from build123d import *

# Parameters (mm, degrees)
SKETCH1_W           = 157.13579329
SKETCH1_H           = 157.13579329
BOSS_EXTRUDE1_DEPTH = 25.4
SKETCH2_W           = 136.81579329
SKETCH2_H           = 111.41579329
CUT_EXTRUDE1_DEPTH  = 22.86
SKETCH3_W           = 136.81579329
SKETCH3_H           = 25.4
CUT_EXTRUDE2_DEPTH  = 22.86
SKETCH5_W           = 5.08
SKETCH5_H           = 136.81579329
CUT_EXTRUDE3_DEPTH  = 7.62
SKETCH6_W           = 8.486375486
SKETCH6_H           = 6.062880986
CUT_EXTRUDE4_DEPTH  = 15.24
SKETCH8_R           = 15.547206761
BOSS_EXTRUDE3_DEPTH = 17.78


with BuildPart() as part:
    # Sketch1 → Boss-Extrude1 (new body)
    with BuildSketch(Plane.XY):
        Rectangle(SKETCH1_W, SKETCH1_H)
    extrude(amount=BOSS_EXTRUDE1_DEPTH)

    # Sketch2 → Cut-Extrude1 (cut)
    with BuildSketch(Plane.XY.offset(25.4)):
        with Locations((0, 12.7)):
            Rectangle(SKETCH2_W, SKETCH2_H)
    extrude(amount=-CUT_EXTRUDE1_DEPTH, mode=Mode.SUBTRACT)

    # Sketch3 → Cut-Extrude2 (cut)
    with BuildSketch(Plane.XY.offset(25.4)):
        with Locations((0, -60.787896645)):
            Rectangle(SKETCH3_W, SKETCH3_H)
    extrude(amount=-CUT_EXTRUDE2_DEPTH, mode=Mode.SUBTRACT)

    # Sketch5 → Cut-Extrude3 (cut)
    with BuildSketch(Plane.ZY.offset(78.567896645)):
        with Locations((12.7, 0)):
            Rectangle(SKETCH5_W, SKETCH5_H)
    cut_extrude3 = extrude(amount=-CUT_EXTRUDE3_DEPTH, mode=Mode.SUBTRACT)

    # Mirror1: Cut-Extrude3 across plane
    add(cut_extrude3.mirror(Plane(origin=(0, 0, 0), x_dir=(0, 0, 1), z_dir=(1, 0, 0))), mode=Mode.SUBTRACT)

    # Sketch6 → Cut-Extrude4 (cut)
    with BuildSketch(Plane.XY.offset(25.4)):
        with Locations((-51.293944562, 71.439337138)):
            Rectangle(SKETCH6_W, SKETCH6_H)
    extrude(amount=-CUT_EXTRUDE4_DEPTH, mode=Mode.SUBTRACT)

    # Sketch8 → Boss-Extrude3 (add)
    with BuildSketch(Plane.XY.offset(2.54)):
        with Locations((39.391283746, 8.898945532)):
            Circle(SKETCH8_R)
    extrude(amount=BOSS_EXTRUDE3_DEPTH)


solid = part.part
Verification items for the finished model (mm, model axes). A direction names the side the tool comes from. Round coordinates to 2 decimals unless told otherwise and drop trailing zeros. Loops run counter-clockwise (first coordinate to the right, second up) from the corner with the lowest first, then second, coordinate; pieces in that order, holes last. Notation, with made-up numbers: (43.25, 37.5) - (53.25, 37.5) arc R36 ccw to (53.25, 71.5) - close; hole circle Ø3 at (-10.5, -9.5). An arc over 180 degrees is marked (long way). Answer in a Markdown table with one row per item. Add a question column.
Q1. Gauge pin test, flat ends, axial feed: pin 1 (10 mm diameter, centred on x = 13.5, y = -24.5, fed in from +Z); pin 2 (15.5 mm diameter, centred on x = 41.5, y = 2.5, fed in from +Z). Record the tip position at first contact, or that the pin passes through.
Q2. Release check for a two-part mould opening along Z. For faces 4 (the face through (-1, -78.568, 13)), 5 (the face through (-1, 13, 2.54)), 6 (the face through (75, -1, 15.24)), 7 (the face through (-75, -1, 10.16)) record: pulls with the +Z half, pulls with the -Z half, needs draft (parallel to the pull), parting line crosses it, or undercut.
Q3. Section check C-C on y = -45. Enter the section's corners in (x, z), plus the area to 3 significant figures.
Q4. Section check B-B on x = -49. Enter the section's corners in (y, z), plus the area to 3 significant figures.
Q5. Section check D-D on y = 38. Enter the section's corners in (x, z), plus the area to 3 significant figures.
Q6. Material ranges on line 1 (Y direction, x = 17, z = 8.75); line 2 (X direction, y = -58, z = 18.75); line 3 (X direction, y = 14.5, z = 15), recorded low to high.
Q7. Section check A-A on z = 17.75. Enter the section's corners in (x, y), plus the area to 3 significant figures.
Q8. Tool access check on faces 1 (the face through (68.408, -61, 14)), 2 (the face through (-75, -68.408, 13)), 3 (the face through (70.948, 1, 13)). Record the directions out of +Z, -Z, +X, -X, +Y, -Y that give a thin tool (end or side, any length) a straight path to the whole face; none if there is none.
Found:
| question | item | result |
|---|---|---|
| 1 | pin 1 | stops at z = 2.54 |
| 1 | pin 2 | stops at z = 20.32 |
| 2 | face 4 | needs draft |
| 2 | face 5 | pulls with the +Z half |
| 2 | face 6 | undercut |
| 2 | face 7 | undercut |
| 3 | outline | (-78.57, 0) - (78.57, 0) - (78.57, 10.16) - (70.95, 10.16) - (70.95, 15.24) - (78.57, 15.24) - (78.57, 25.4) - (-78.57, 25.4) - (-78.57, 15.24) - (-70.95, 15.24) - (-70.95, 10.16) - (-78.57, 10.16) - close |
| 3 | area | 3,910 mm² |
| 4 | outline | (-78.57, 0) - (78.57, 0) - (78.57, 25.4) - (74.47, 25.4) - (74.47, 10.16) - (68.41, 10.16) - (68.41, 2.54) - (-43.01, 2.54) - (-43.01, 25.4) - (-48.09, 25.4) - (-48.09, 2.54) - (-73.49, 2.54) - (-73.49, 25.4) - (-78.57, 25.4) - close |
| 4 | area | 771 mm² |
| 5 | outline | (-78.57, 0) - (78.57, 0) - (78.57, 10.16) - (70.95, 10.16) - (70.95, 15.24) - (78.57, 15.24) - (78.57, 25.4) - (68.41, 25.4) - (68.41, 2.54) - (-68.41, 2.54) - (-68.41, 25.4) - (-78.57, 25.4) - (-78.57, 15.24) - (-70.95, 15.24) - (-70.95, 10.16) - (-78.57, 10.16) - close |
| 5 | area | 786 mm² |
| 6 | line 1 | y = -78.57 to -73.49, -48.09 to -43.01, 68.41 to 78.57 |
| 6 | line 2 | x = -78.57 to -68.41, 68.41 to 78.57 |
| 6 | line 3 | x = -70.95 to -68.41, 24.89 to 53.89, 68.41 to 70.95 |
| 7 | outline | (-78.57, -78.57) - (78.57, -78.57) - (78.57, 78.57) - (-78.57, 78.57) - close; circle Ø31.09 at (39.39, 8.9); hole (-68.41, -73.49) - (68.41, -73.49) - (68.41, -48.09) - (-68.41, -48.09) - close; hole (-68.41, -43.01) - (68.41, -43.01) - (68.41, 68.41) - (-47.05, 68.41) - (-47.05, 74.47) - (-55.54, 74.47) - (-55.54, 68.41) - (-68.41, 68.41) - close |
| 7 | area | 6,680 mm² |
| 8 | face 1 | +Z |
| 8 | face 2 | -X |
| 8 | face 3 | +X |
